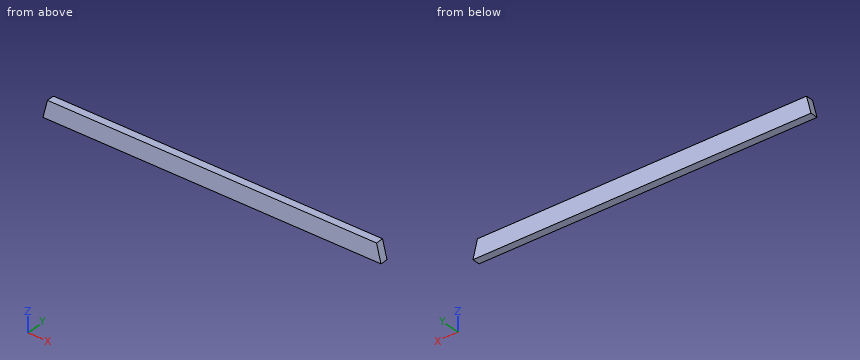
from build123d import *

# Parameters (mm, degrees)
F0_W     = 38.1
F0_H     = 88.9
F1_DEPTH = 842.9625
F2_SIZE2 = 88.89999
F2_SIZE  = 22.22499


# Not quite as in the source:
# - a fillet or chamfer is up to 0.001 mm smaller than in the source, because OpenCascade refuses the exact size


with BuildPart() as f1:
    # F0 (on Right) → F1 (new body, symmetric)
    with BuildSketch(Plane.YZ):
        Rectangle(F0_W, F0_H)
    extrude(amount=F1_DEPTH, both=True)

    # F2 (size 22.225 and 88.9 in the source; OpenCascade refuses exactly that, so slightly less here)
    f2_edges = [f1.edges().sort_by_distance(p)[0] for p in [
        (842.9625, 0, 44.45),
        (-842.9625, 0, 44.45),
    ]]
    f2_side = f1.faces().sort_by_distance((0, 0, 44.45))[0]
    chamfer(f2_edges, length=F2_SIZE, length2=F2_SIZE2, reference=f2_side)


solid = f1.part
The model under review builds one solid part; all positions refer to its coordinate system, in mm. Round coordinates to 2 decimals unless told otherwise and drop trailing zeros. Write each loop counter-clockwise with the first axis right and the second up, starting at its lowest first coordinate (ties: lowest second). Pieces come first, ordered by that corner, then holes. Notation, with made-up numbers: M 42,-7 L 80,-7 A18 cw 80,2 Z; hole C 6.25,87.25 d11. An arc over 180 degrees is marked long. Use a Markdown table: item, result. Add a question column.
Q1. Insertion check: pin 1 (4 mm diameter, centred on y = -7.5, z = 17, fed in from +X); pin 2 (3 mm diameter, centred on y = -2, z = -31.5, fed in from -X); pin 3 (8 mm diameter, centred on y = -5.5, z = -27, fed in from +X). Each pin has a flat end and moves straight along its axis. Give the tip position at first contact, or say it passes through.
Q2. We need section A-A, the plane z = 9. State the section outline as (x, y) points, plus the area to 3 significant figures.
Q3. To check wall thickness, follow line 1 (X direction, y = 7, z = -7); line 2 (X direction, y = -11, z = -40). State the ranges of each line that lie inside material, in increasing order.
Findings below:
| question | item | result |
|---|---|---|
| 1 | pin 1 | stops at x = 828.1 |
| 1 | pin 2 | stops at x = -840.1 |
| 1 | pin 3 | stops at x = 839.6 |
| 2 | outline | M -829.6,-19.05 L 829.6,-19.05 L 829.6,19.05 L -829.6,19.05 Z |
| 2 | area | 63,200 mm² |
| 3 | line 1 | x = -833.6 to 833.6 |
| 3 | line 2 | x = -841.85 to 841.85 |
